Source: CAD feature listing. Evaluate the final solid. Frame: model axes, mm. Face numbers are marked on the shaded views. A direction names the side the tool comes from. Round coordinates to 2 decimals unless told otherwise and drop trailing zeros. Order: outer loops, then holes, each group sorted by start corner. A loop starts at its lowest first (then second) coordinate and runs counter-clockwise, first axis right, second up. Notation, with made-up numbers: (-29, 63) -> (17, 63) arc R14 cw to (17, 85) -> close; hole circle Ø7 at (-4.5, -11.5). An arc over 180 degrees is marked (long way). Write item = value, one per line. Start each with the question number.
(1) Cut plane A-A on z = 0. Return the cut outline in (x, y), then the cut area to 3 significant figures.
(2) Contact query for flat-ended pins moving along their axis: pin 1 Ø4.5 at (x, z) = (-5, -1.5) entering from -Y; pin 2 Ø0.5 at (x, y) = (2, -2) entering from -Z; pin 3 Ø2.5 at (y, z) = (12, -0.5) entering from +X. Output: stop coordinate, or through.
(3) Cut plane C-C on y = 4.75. Return the cut outline in (x, z), then the cut area to 3 significant figures.
(4) Cut plane B-B on y = 1.25. Return the cut outline in (x, z), then the cut area to 3 significant figures.
(5) Ray query, line 1 (X direction, y = 11.25, z = -0.25); line 2 (Y direction, x = -2, z = -2); line 3 (Y direction, x = -2.75, z = -5.5). Return the intervals inside material, ascending.
(6) Reachability of the marked faces 1, 2 and 3 from +Z, -Z, +X, -X, +Y, -Y: full face, straight path, thin tool, end or side. Return the list, or none.
from build123d import *
from build123d.topology import SkipClean

# Parameters (mm, degrees)
SKETCH1_R            = 6.5
BOSS_EXTRUDE1_DEPTH  = 3.1
SKETCH2_R            = 4
BOSS_EXTRUDE2_DEPTH  = 0.5
SKETCH3_R            = 2.4
BOSS_EXTRUDE3_DEPTH  = 3
SKETCH4_R            = 1.7
BOSS_EXTRUDE4_DEPTH  = 6.8
CHAMFER1_SIZE        = 0.15
CUT_EXTRUDE1_DEPTH   = 4.5
SKETCH6_R            = 6.4
BOSS_EXTRUDE5_DEPTH  = 1
FILLET1_R            = 0.4
CHAMFER2_SIZE        = 0.1
BOSS_EXTRUDE6_DEPTH  = 1.2
SKETCH8_W            = 1.400599112
SKETCH8_H            = 0.2
BOSS_EXTRUDE7_DEPTH  = 1.2
SKETCH9_W            = 1.400599112
SKETCH9_H            = 0.2
BOSS_EXTRUDE8_DEPTH  = 1.2
SKETCH10_W           = 1.370501576
SKETCH10_H           = 0.2
BOSS_EXTRUDE9_DEPTH  = 1.2
FILLET2_R            = 0.5
FILLET3_R            = 0.2
SKETCH11_W           = 1.09784978
SKETCH11_H           = 0.766423431
SKETCH11_W_2         = 1.035707339
SKETCH11_H_2         = 0.70428099
SKETCH11_W_3         = 1.242848807
BOSS_EXTRUDE10_DEPTH = 2


with BuildPart() as part:
    # Sketch1 → Boss-Extrude1 (new body)
    with BuildSketch(Plane(origin=(0, 0, 0), x_dir=(1, 0, 0), z_dir=(0, 1, 0))):
        with Locations(Location((0, 0, 0), (0, 0, 90))):
            Circle(SKETCH1_R)
    extrude(amount=BOSS_EXTRUDE1_DEPTH)

    # Sketch2 → Boss-Extrude2 (add)
    with BuildSketch(Plane(origin=(0, 3.1, 0), x_dir=(1, 0, 0), z_dir=(0, 1, 0))):
        with Locations(Location((0, 0, 0), (0, 0, 270))):
            Circle(SKETCH2_R)
    extrude(amount=BOSS_EXTRUDE2_DEPTH)

    # Sketch3 → Boss-Extrude3 (add)
    with BuildSketch(Plane(origin=(0, 3.6, 0), x_dir=(-1, 0, 0), z_dir=(0, 1, 0))):
        with Locations(Location((0, 0, 0), (0, 0, 90))):
            Circle(SKETCH3_R)
    extrude(amount=BOSS_EXTRUDE3_DEPTH)

    # Sketch4 → Boss-Extrude4 (add)
    with BuildSketch(Plane(origin=(0, 6.6, 0), x_dir=(1, 0, 0), z_dir=(0, 1, 0))):
        with Locations(Location((0, 0, 0), (0, 0, 270))):
            Circle(SKETCH4_R)
    extrude(amount=BOSS_EXTRUDE4_DEPTH)

    # Chamfer1
    chamfer1_edges = [part.edges().sort_by_distance(p)[0] for p in [
        (0, 13.4, -1.7),
    ]]
    chamfer(chamfer1_edges, length=CHAMFER1_SIZE)

    # Sketch5 → Cut-Extrude1 (cut)
    with BuildSketch(Plane(origin=(0, 13.4, 0), x_dir=(1, 0, 0), z_dir=(0, 1, 0))):
        Polygon((0.95, 0), (0.95, 1.953547683), (2.291589772, 1.953547683), (2.291589772, -1.88704126), (0.95, -1.88704126), align=None)
        Polygon((-0.95, 0), (-0.95, 2.055691006), (-2.284431096, 2.055691006), (-2.21293077, -1.815540934), (-0.95, -1.815540934), align=None)
    extrude(amount=-CUT_EXTRUDE1_DEPTH, mode=Mode.SUBTRACT)

    # Sketch6 → Boss-Extrude5 (add)
    with BuildSketch(Plane.XZ):
        with Locations(Location((0, 0, 0), (0, 0, 90))):
            Circle(SKETCH6_R)
    extrude(amount=BOSS_EXTRUDE5_DEPTH)

    # Fillet1
    fillet1_edges = [part.edges().sort_by_distance(p)[0] for p in [
        (0, 3.1, 6.5),
    ]]
    fillet(fillet1_edges, radius=FILLET1_R)

    # Chamfer2
    chamfer2_edges = [part.edges().sort_by_distance(p)[0] for p in [
        (0, 6.6, -2.4),
    ]]
    chamfer(chamfer2_edges, length=CHAMFER2_SIZE)

    # Sketch7 → Boss-Extrude6 (add)
    with SkipClean():  # the faces are left unmerged after this step: merging them gives an invalid solid
        with BuildSketch(Plane.XZ):
            with BuildLine():
                Line((5.151524141, 3.79760438), (5.242126256, 3.843190382))
                ThreePointArc((5.242126256, 3.843190382), (5.626855667, 3.253996819), (5.945638893, 2.626666738))
                Line((5.945638893, 2.626666738), (5.854255539, 2.586057247))
                Line((5.854255539, 2.586057247), (5.151524141, 3.79760438))
            make_face()
            with BuildLine():
                Line((-5.242126256, 3.843190382), (-5.151524141, 3.79760438))
                Line((-5.151524141, 3.79760438), (-5.854255539, 2.586057247))
                Line((-5.854255539, 2.586057247), (-5.945638893, 2.626666738))
                ThreePointArc((-5.945638893, 2.626666738), (-5.626855667, 3.253996819), (-5.242126256, 3.843190382))
            make_face()
            with BuildLine():
                Line((-0.7, -6.462197769), (-0.688624102, -6.362845028))
                Line((-0.688624102, -6.362845028), (0.681877282, -6.363571589))
                Line((0.681877282, -6.363571589), (0.7, -6.462197769))
                ThreePointArc((0.7, -6.462197769), (0, -6.5), (-0.7, -6.462197769))
            make_face()
        extrude(amount=BOSS_EXTRUDE6_DEPTH)

    # Sketch8 → Boss-Extrude7 (add)
    with SkipClean():  # the faces are left unmerged after this step: merging them gives an invalid solid
        with BuildSketch(Plane(origin=(5.50288984, 0, 3.191830814), x_dir=(-0.5017362869920535, 0, 0.8650206346182893), z_dir=(-0.8650206346182893, 0, -0.5017362869920535))):
            with Locations((0, -1.1)):
                Rectangle(SKETCH8_W, SKETCH8_H)
        extrude(amount=BOSS_EXTRUDE7_DEPTH)

    # Sketch9 → Boss-Extrude8 (add)
    with SkipClean():  # the faces are left unmerged after this step: merging them gives an invalid solid
        with BuildSketch(Plane(origin=(-5.50288984, 0, 3.191830814), x_dir=(-0.5017362869920535, 0, -0.8650206346182893), z_dir=(0.8650206346182893, 0, -0.5017362869920535))):
            with Locations((0, -1.1)):
                Rectangle(SKETCH9_W, SKETCH9_H)
        extrude(amount=BOSS_EXTRUDE8_DEPTH)

    # Sketch10 → Boss-Extrude9 (add)
    with SkipClean():  # the faces are left unmerged after this step: merging them gives an invalid solid
        with BuildSketch(Plane(origin=(-0.00337341, 0, -6.363208308), x_dir=(0.9999998594742814, 0, -0.0005301428274771333), z_dir=(0.0005301428274771333, 0, 0.9999998594742814))):
            with Locations((0, -1.1)):
                Rectangle(SKETCH10_W, SKETCH10_H)
        extrude(amount=BOSS_EXTRUDE9_DEPTH)

    # Fillet2
    fillet2_edges = [part.edges().sort_by_distance(p)[0] for p in [
        (4.113499379, -1.1, 3.195520836),
        (4.816230777, -1.1, 1.983973703),
        (-4.113499379, -1.1, 3.195520836),
        (-4.816230777, -1.1, 1.983973703),
        (0.682513454, -1.1, -5.163571758),
        (-0.68798793, -1.1, -5.162845196),
    ]]
    fillet(fillet2_edges, radius=FILLET2_R)

    # Fillet3
    fillet3_edges = [part.edges().sort_by_distance(p)[0] for p in [
        (5.626855667, -1.2, 3.253996819),
        (0, -1.2, -6.5),
        (-5.626855667, -1.2, 3.253996819),
    ]]
    fillet(fillet3_edges, radius=FILLET3_R)

    # Sketch11 → Boss-Extrude10 (add)
    with BuildSketch(Plane.XZ.offset(1)):
        with Locations((-0.051193187, 1.87960604)):
            Rectangle(SKETCH11_W, SKETCH11_H)
        with Locations((1.947721978, 2.967098746)):
            Rectangle(SKETCH11_W_2, SKETCH11_H_2)
        with Locations((-2.505819581, 2.967098746)):
            Rectangle(SKETCH11_W_3, SKETCH11_H_2)
    extrude(amount=BOSS_EXTRUDE10_DEPTH)


solid = part.part
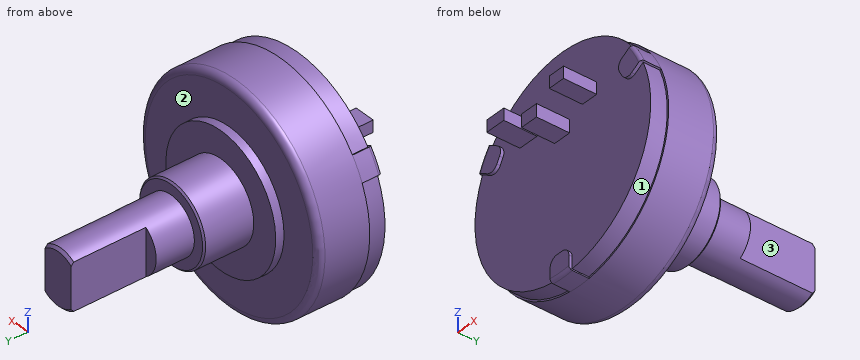
Evaluation:
q1.outline = (-6.5, 0) -> (-6.4, 0) -> (-6.4, -1) -> (6.4, -1) -> (6.4, 0) -> (6.5, 0) -> (6.5, 2.7) arc R0.4 ccw to (6.1, 3.1) -> (4, 3.1) -> (4, 3.6) -> (2.4, 3.6) -> (2.4, 6.5) -> (2.3, 6.6) -> (1.7, 6.6) -> (1.7, 8.9) -> (0.95, 8.9) -> (0.95, 13.4) -> (-0.95, 13.4) -> (-0.95, 8.9) -> (-1.7, 8.9) -> (-1.7, 6.6) -> (-2.3, 6.6) -> (-2.4, 6.5) -> (-2.4, 3.6) -> (-4, 3.6) -> (-4, 3.1) -> (-6.1, 3.1) arc R0.4 ccw to (-6.5, 2.7) -> close
q1.area = 87.8 mm^2
q2.pin_1 = -1
q2.pin_2 = 2.61
q2.pin_3 = 0.95
q3.outline = circle Ø4.8 at (0, 0)
q3.area = 18.1 mm^2
q4.outline = circle Ø13 at (0, 0)
q4.area = 133 mm^2
q5.line_1 = -0.95 to 0.95
q5.line_2 = -1 to 3.6
q5.line_3 = -1 to 3.1
q6.face_1 = +X, -Y
q6.face_2 = +Y
q6.face_3 = +Z, -Z, +X, +Y
